Could you check a few things on this model? Use its own coordinates, in mm. Give positions to 0.01 mm unless a question says otherwise; leave off trailing zeros. Order: outer loops, then holes, each group sorted by start corner. A loop starts at its lowest first (then second) coordinate and runs counter-clockwise, first axis right, second up. Notation, with made-up numbers: M 31,15 L 90,15 A21 ccw 90,51 Z; hole C 67,5.5 d3. An arc over 180 degrees is marked long. Use a Markdown table: item, result. Add a question column.
Item 1: Suppose I cut it at A-A on x = -4.75. Write out the boundary of the cut face in (y, z), plus the area to 3 significant figures.
Item 2: I'm going to push a flat-ended pin straight in: pin 1 Ø3 at (x, y) = (0, 1.5) entering from -Z. Where does the tip first touch, or does it pass through?
Item 3: Suppose I cut it at B-B on y = -1.9. Write out the boundary of the cut face in (x, z).
Item 4: If I drill on L1, parallel to Y at x = -3.05, z = 5.75; L2, parallel to Y at x = 4.75, z = 3.5; L3, parallel to Y at x = -4.75, z = 0.75, over which ranges is the centre line in solid material (lowest first)? Write a range as from..to.
Item 5: Suppose I cut it at C-C on z = 1.75. Write out the boundary of the cut face in (x, y), plus the area to 3 significant figures.
Item 6: Suppose I cut it at D-D on x = -3.05. Write out the boundary of the cut face in (y, z).
from build123d import *

# Parameters (mm, degrees)
F0_W     = 13.5
F0_H     = 7.8
F0_R     = 0.4
F1_DEPTH = 8


with BuildPart() as f1:
    # F0 (on Top) → F1 (new body)
    with BuildSketch(Plane.XY):
        Rectangle(F0_W, F0_H)
        with Locations((-3.05, -1.9)):
            Circle(F0_R, mode=Mode.SUBTRACT)
        with Locations((4.75, -1.27)):
            Circle(F0_R, mode=Mode.SUBTRACT)
        with Locations((-4.75, 1.9)):
            Circle(F0_R, mode=Mode.SUBTRACT)
        with Locations((-3.05, 1.9)):
            Circle(F0_R, mode=Mode.SUBTRACT)
        with Locations((4.75, 1.27)):
            Circle(F0_R, mode=Mode.SUBTRACT)
    extrude(amount=F1_DEPTH)


solid = f1.part
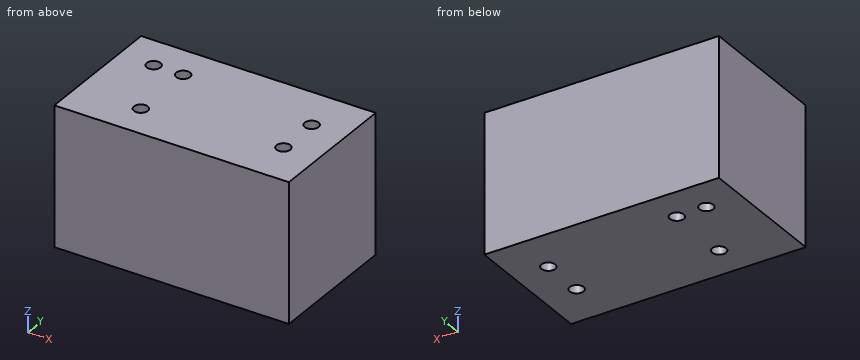
Findings below:
| question | item | result |
|---|---|---|
| 1 | outline | M -3.9,0 L 1.5,0 L 1.5,8 L -3.9,8 Z; M 2.3,0 L 3.9,0 L 3.9,8 L 2.3,8 Z |
| 1 | area | 56.0 mm^2 |
| 2 | pin 1 | stops at z = 0 |
| 3 | outline | M -6.75,0 L -3.45,0 L -3.45,8 L -6.75,8 Z; M -2.65,0 L 6.75,0 L 6.75,8 L -2.65,8 Z |
| 4 | L1 | y = -3.9..-2.3, -1.5..1.5, 2.3..3.9 |
| 4 | L2 | y = -3.9..-1.67, -0.87..0.87, 1.67..3.9 |
| 4 | L3 | y = -3.9..1.5, 2.3..3.9 |
| 5 | outline | M -6.75,-3.9 L 6.75,-3.9 L 6.75,3.9 L -6.75,3.9 Z; hole C -4.75,1.9 d0.8; hole C -3.05,-1.9 d0.8; hole C -3.05,1.9 d0.8; hole C 4.75,-1.27 d0.8; hole C 4.75,1.27 d0.8 |
| 5 | area | 103 mm^2 |
| 6 | outline | M -3.9,0 L -2.3,0 L -2.3,8 L -3.9,8 Z; M -1.5,0 L 1.5,0 L 1.5,8 L -1.5,8 Z; M 2.3,0 L 3.9,0 L 3.9,8 L 2.3,8 Z |
